Answer from the drawing. Dimensions are ordinates in mm from the lowest x, y and z of the part. Give positions to 0.01 mm unless a question says otherwise; leave off trailing zeros. Write each question's results on one line, items separated by ' | '. Start each with the question number.
Item 1: Find the intervals of material crossed by line 1 (Z direction, x = 18.3, y = 1.05); line 2 (Y direction, x = 16, z = 9.25) (1 decimal); line 3 (Z direction, x = 13.75, y = 0.9), in increasing order.
Item 2: Section B-B on z = 13.5 is taken. State how many separate pieces and enclosed holes the cut face has.
Item 3: Each of these flat-tipped pins is pushed along its axis until it touches: P1, Ø1, axis at x = 3, y = 2.5, coming from the -Z side; P2, Ø2, axis at x = 10, z = 9.5, coming from the +Y side; P3, Ø0.6, axis at x = 10, y = 2.5, coming from the -Z side; P4, Ø0.5, axis at y = 3, z = 13.5, coming from the +X side. Where does it stop, or does it pass through?
Item 4: Determine the mould class of the marked faces 1, 2 and 3 for opening direction Z: +Z half, -Z half, draft (parallel to the pull), parting line (faces both ways), or undercut.
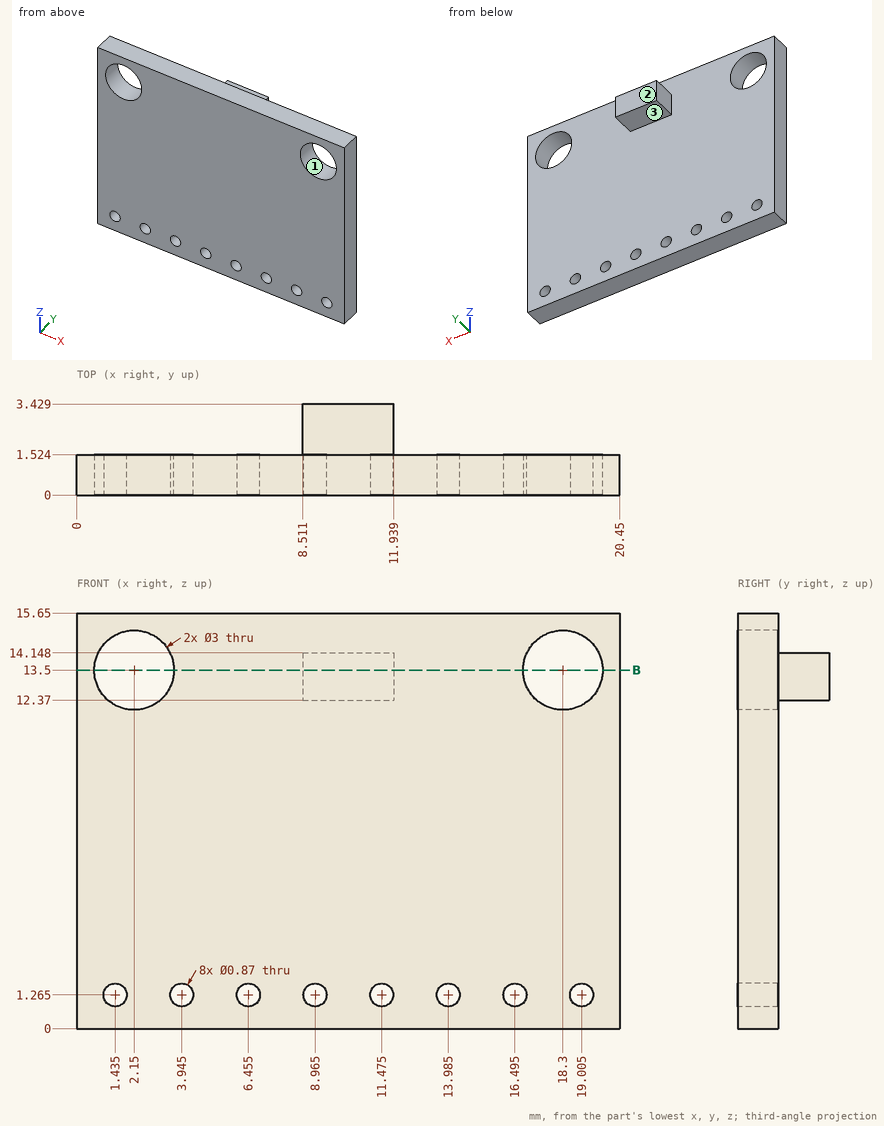
Findings:
1) line 1: 0 to 12, 15 to 15.65 | line 2: 0 to 1.5 | line 3: 0 to 0.9, 1.63 to 15.65
2) separate pieces: 3 | enclosed holes: 0
3) P1: through | P2: y = 1.52 | P3: z = 12.37 | P4: x = 11.94
4) face 1: undercut | face 2: draft | face 3: -Z half
